Read the model definition and answer for the solid it produces. Units are mm, in the model's axes. Coordinates: 2 decimals unless noted, no trailing zeros. Loops run counter-clockwise (first coordinate to the right, second up) from the corner with the lowest first, then second, coordinate; pieces in that order, holes last.
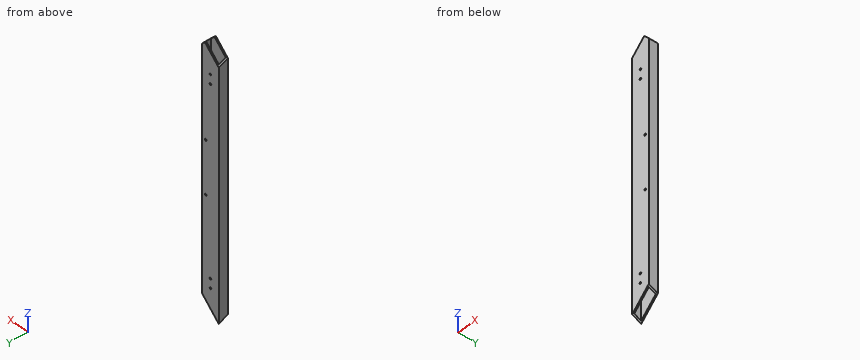
from build123d import *

# Parameters (mm, degrees)
SKETCH1_W                        = 50.8
SKETCH1_H                        = 25.4
SKETCH1_W_2                      = 44.45
SKETCH1_H_2                      = 19.05
BOSS_EXTRUDE1_DEPTH              = 771.9314
CUT_EXTRUDE1_DEPTH               = 771.9314
CUT_EXTRUDE2_DEPTH               = 773.76672179
CUT_EXTRUDE3_DEPTH               = 757.919388013
CUT_EXTRUDE5_DEPTH               = 771.9314
SKETCH7_R                        = 2.4638
CUT_EXTRUDE6_DEPTH               = 730.251464289
SKETCH8_R                        = 2.4638
CUT_EXTRUDE7_DEPTH               = 730.251464289
F_13_64_0_20313_DIAMETER_HOLE1_D = 5.159502


with BuildPart() as part:
    # Sketch1 → Boss-Extrude1 (new body)
    with BuildSketch(Plane.XY):
        Rectangle(SKETCH1_W, SKETCH1_H)
        Rectangle(SKETCH1_W_2, SKETCH1_H_2, mode=Mode.SUBTRACT)
    extrude(amount=BOSS_EXTRUDE1_DEPTH)

    # Sketch2 → Cut-Extrude1 (cut)
    with BuildSketch(Plane(origin=(0, 12.7, 0), x_dir=(1, 0, 0), z_dir=(0, 1, 0))):
        Polygon((-25.4, 0), (25.4, -50.8), (25.4, 0), align=None)
        Polygon((25.4, -771.9314), (-25.4, -721.1314), (-25.4, -771.9314), align=None)
    extrude(amount=-CUT_EXTRUDE1_DEPTH, mode=Mode.SUBTRACT)

    # Sketch3 → Cut-Extrude2 (cut, through all)
    with BuildSketch(Plane(origin=(0, 12.7, 0), x_dir=(1, 0, 0), z_dir=(0, 1, 0))):
        Polygon((-3.3782, -743.1532), (25.4, -714.375), (25.4, -771.9314), (-3.3782, -771.9314), align=None)
    extrude(amount=-CUT_EXTRUDE2_DEPTH, mode=Mode.SUBTRACT)

    # Sketch4 → Cut-Extrude3 (cut, through all)
    with BuildSketch(Plane(origin=(-12.7, 0, -12.7), x_dir=(0, -1, 0), z_dir=(0.7071067811865571, 0, 0.707106781186538))):
        Polygon((-12.7, -17.960512242), (12.7, -26.213472526), (12.7, -17.960512242), align=None)
    extrude(amount=CUT_EXTRUDE3_DEPTH, mode=Mode.SUBTRACT)

    # Sketch6 → Cut-Extrude5 (cut)
    with BuildSketch(Plane(origin=(369.8875, 0, 369.8875), x_dir=(0.7071067811865437, 0, -0.7071067811865513), z_dir=(0.7071067811865513, 0, 0.7071067811865437))):
        Polygon((-506.965494568, -12.7), (-498.712534284, 12.7), (-506.965494568, 12.7), (-527.877415309, 12.7), (-527.877415309, -12.7), align=None)
    extrude(amount=-CUT_EXTRUDE5_DEPTH, mode=Mode.SUBTRACT)

    # Sketch7 → Cut-Extrude6 (cut, through all)
    with BuildSketch(Plane.XZ.offset(12.7)):
        with Locations(Location((0, 105.257676555, 0), (0, 0, 270))):
            Circle(SKETCH7_R)
        with Locations(Location((0, 79.857676555, 0), (0, 0, 270))):
            Circle(SKETCH7_R)
    extrude(amount=-CUT_EXTRUDE6_DEPTH, mode=Mode.SUBTRACT)

    # Sketch8 → Cut-Extrude7 (cut, through all)
    with BuildSketch(Plane(origin=(0, 12.7, 0), x_dir=(1, 0, 0), z_dir=(0, 1, 0))):
        with Locations(Location((0, -646.867704494, 0), (0, 0, 270))):
            Circle(SKETCH8_R)
        with Locations(Location((0, -621.467704494, 0), (0, 0, 270))):
            Circle(SKETCH8_R)
    extrude(amount=-CUT_EXTRUDE7_DEPTH, mode=Mode.SUBTRACT)

    # 13/64 (0.20313) Diameter Hole1 (through all)
    with Locations(Plane(origin=(0, -12.7, 0), x_dir=(-1, 0, 0), z_dir=(0, -1, 0))):
        with Locations((-14.2367, -319.172239037), (-14.2367, -464.968239037)):
            Hole(F_13_64_0_20313_DIAMETER_HOLE1_D / 2)


solid = part.part
Q1. A cutting plane is placed at A-A (z = 188). Give the vertices of the cut face in (x, y) (3 decimals).
Findings below:
outline: (-25.4, -12.7) - (25.4, -12.7) - (25.4, 12.7) - (-25.4, 12.7) - close; hole (-22.225, -9.525) - (22.225, -9.525) - (22.225, 9.525) - (-22.225, 9.525) - close
Q2. Flat-ended cylindrical pins translate along their axes: pin 1 Ø4.5 at (x, z) = (0, 646.87) entering from +Y; pin 2 Ø6 at (x, y) = (9, 7) entering from +Z. Find the tip coordinate at first contact, or state that the pin passes through.
Findings below:
pin 1: passes through
pin 2: stops at z = 717.36
Q3. A cutting plane is placed at B-B (y = 0.5). Give the vertices of the cut face in (x, z) (3 decimals), then the cut area to 3 significant figures.
Findings below:
outline: (-25.4, 5.606) - (-22.225, 8.781) - (-22.225, 688.667) - (-25.4, 685.492) - close; (22.225, 53.231) - (25.4, 56.406) - (25.4, 714.375) - (22.225, 717.55) - close
area: 4,260 mm2
Q4. Straight lines are drawn through the part: probe 1 along X at (y, z) = (2.75, 400) (3 decimals); probe 2 along Y at (x, z) = (21.5, 569.5) (3 decimals); probe 3 along Z at (x, y) = (16.5, 10.75). For each, find the intervals that lie inside material, in ascending order.
Findings below:
probe 1: x = -25.4 to -22.225, 22.225 to 25.4
probe 2: y = -12.7 to -9.525, 9.525 to 12.7
probe 3: z = 42.8 to 317.93, 320.41 to 463.73, 466.21 to 722.68
